Read the model definition and answer for the solid it produces. Units are mm, in the model's axes. A direction names the side the tool comes from. Give positions to 0.01 mm unless a question says otherwise; leave off trailing zeros. Order: outer loops, then holes, each group sorted by start corner. A loop starts at its lowest first (then second) coordinate and runs counter-clockwise, first axis right, second up. Notation, with made-up numbers: (-6.75, -8) -> (18.25, -8) arc R16 cw to (18.25, 0) -> close; hole circle Ø5 at (-2, -26). An arc over 180 degrees is marked (long way). One line per question, with ' | ' between items. Start each with the question number.
```python
from build123d import *

# Parameters (mm, degrees)
POCKET_DEPTH       = 76.251136
POCKET_DEPTH_BACK  = 76.251136
POLARPATTERN_COUNT = 18
CHAMFER_SIZE       = 0.5


with BuildPart() as part:
    # Sketch → Revolution (revolve)
    with BuildSketch(Plane.XZ):
        Polygon((-7.55, 7.15), (-7.05, 7.15), (-7.05, 8.25), (-7.55, 8.25), (-7.55, 12), (-4.05, 12), (-4.05, -12), (-7.55, -12), (-7.55, -8.25), (-7.05, -8.25), (-7.05, -7.15), (-7.55, -7.15), align=None)
    revolve(axis=Axis((0, 0, 0), (0, 0, 1)))

    # Sketch001 → Pocket (cut, two sides)
    with BuildSketch(Plane.XY) as pocket_sk:
        with BuildLine():
            Line((0, 0), (-0.479357, 5.479071))
            ThreePointArc((0.479357, 5.479071), (0, 5.5), (-0.479357, 5.479071))
            Line((0.479357, 5.479071), (0, 0))
        make_face()
    pocket = extrude(amount=-POCKET_DEPTH, mode=Mode.SUBTRACT) + extrude(pocket_sk.sketch, amount=POCKET_DEPTH_BACK, mode=Mode.SUBTRACT)

    # PolarPattern: Pocket ×18 about axis
    polarpattern_axis = Axis((0, 0, 0), (0, 0, 1))
    for i in range(1, POLARPATTERN_COUNT):
        add(pocket.rotate(polarpattern_axis, i * 360 / POLARPATTERN_COUNT), mode=Mode.SUBTRACT)

    # Chamfer
    chamfer_edges = [part.edges().sort_by_distance(p)[0] for p in [
        (7.55, 0, 12),
        (7.55, 0, -12),
    ]]
    chamfer(chamfer_edges, length=CHAMFER_SIZE)


solid = part.part
```
Q1. Which of the six approach directions +Z, -Z, +X, -X, +Y, -Y give full straight-line access (tool end or side, diameter ignored) to faces 1 (the flat face through (-3, 3, 0)), 2 (the cylindrical face through (-3.253, 6.255, 7.708))?
Q2. Determine the mould class of faces 3 (the flat face through (-2, 7, 8.25)), 4 (the flat face through (-3, -3, 0)) for opening direction Z: pulls with the +Z half, pulls with the -Z half, needs draft (parallel to the pull), parting line crosses it, or undercut.
Q3. Given P1, Ø1, axis at x = 2.5, z = 8.5, coming from the +Y side; P2, Ø2, axis at x = 2.5, y = 1, coming from the -Z side; P3, Ø1, axis at y = -2, z = 9, coming from the -X side; P4, Ø6, axis at y = -5.5, z = -3, coming from the +X side, each flat-ended and moving along its own axis, determine where each tip first touches the part or whether it passes through.
Q4. Find the intervals of material crossed by line 1 (Y direction, x = 0.25, z = 4.25); line 2 (Y direction, x = -4.75, z = 7.25); line 3 (Y direction, x = 3.5, z = -3.5), in increasing order.
Q5. A cutting plane is placed at B-B, the plane x = 0. Determine the outline of the cut face in (y, z).
Q6. A cutting plane is placed at A-A, the plane y = 0. Determine the outline of the cut face in (x, z), then the cut area to 3 significant figures.
Geometry results:
1) face 1: +Z, -Z | face 2: none
2) face 3: undercut | face 4: needs draft
3) P1: y = 7.28 | P2: through | P3: x = -7.4 | P4: x = 7.12
4) line 1: -7.55 to -5.49, 5.49 to 7.55 | line 2: -5.21 to -2.77, -2.21 to -1.27, -0.42 to 0.42, 1.27 to 2.21, 2.77 to 5.21 | line 3: -6.69 to -4.24, -3.5 to -2.45, 2.45 to 3.5, 4.24 to 6.69
5) outline: (-7.55, -11.5) -> (-7.05, -12) -> (-5.5, -12) -> (-5.5, 12) -> (-7.05, 12) -> (-7.55, 11.5) -> (-7.55, 8.25) -> (-7.05, 8.25) -> (-7.05, 7.15) -> (-7.55, 7.15) -> (-7.55, -7.15) -> (-7.05, -7.15) -> (-7.05, -8.25) -> (-7.55, -8.25) -> close; (5.5, -12) -> (7.05, -12) -> (7.55, -11.5) -> (7.55, -8.25) -> (7.05, -8.25) -> (7.05, -7.15) -> (7.55, -7.15) -> (7.55, 7.15) -> (7.05, 7.15) -> (7.05, 8.25) -> (7.55, 8.25) -> (7.55, 11.5) -> (7.05, 12) -> (5.5, 12) -> close
6) outline: (-7.55, -11.5) -> (-7.05, -12) -> (-4.05, -12) -> (-4.05, 12) -> (-7.05, 12) -> (-7.55, 11.5) -> (-7.55, 8.25) -> (-7.05, 8.25) -> (-7.05, 7.15) -> (-7.55, 7.15) -> (-7.55, -7.15) -> (-7.05, -7.15) -> (-7.05, -8.25) -> (-7.55, -8.25) -> close; (4.05, -12) -> (7.05, -12) -> (7.55, -11.5) -> (7.55, -8.25) -> (7.05, -8.25) -> (7.05, -7.15) -> (7.55, -7.15) -> (7.55, 7.15) -> (7.05, 7.15) -> (7.05, 8.25) -> (7.55, 8.25) -> (7.55, 11.5) -> (7.05, 12) -> (4.05, 12) -> close | area: 165 mm²
